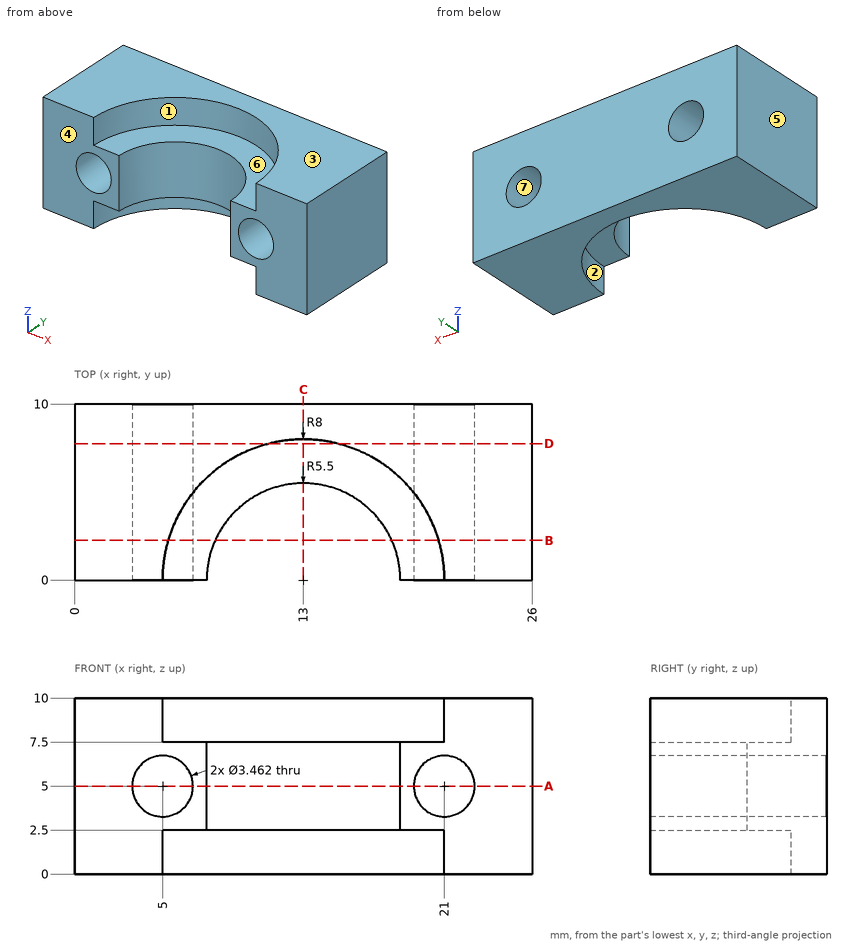
Input: dimensioned drawing with shaded views. Units: mm. Origin: part minimum x, y, z. A direction names the side the tool comes from. Give positions to 0.01 mm unless a question says otherwise; leave off trailing zeros. Write each loop counter-clockwise with the first axis right and the second up, starting at its lowest first coordinate (ties: lowest second). Pieces come first, ordered by that corner, then holes. Notation, with made-up numbers: (14, 72.25) -> (65, 72.25) arc R14 cw to (65, 93.25) -> close; hole circle Ø1 at (-3.5, -35.75). An arc over 180 degrees is marked (long way). Return JSON: item names as keys, results as strings. Group by question number.
1. Section A-A, the plane z = 5. Output: boundary loops of the cut face in (x, y).
2. Pin query (flat end, axial travel): pin 1 Ø2 at (y, z) = (8.5, 7) entering from -X; pin 2 Ø2 at (x, y) = (7.5, 1.5) entering from -Z; pin 3 Ø2 at (x, z) = (15.5, 4.5) entering from -Y. Return the tip coordinate at first contact, or that it passes through.
3. Material intervals for line 1 (Z direction, x = 21, y = 3.25); line 2 (Z direction, x = 7.75, y = 4.75); line 3 (X direction, y = 4, z = 1.25), sorted ascending. Write a range as from..to.
4. Mould query, pull axis X, two halves, no side actions, for the marked faces 4, 5, 6 and 7. Classes: +X half, -X half, draft (parallel to the pull), parting line (faces both ways), or undercut.
5. Access query for the marked faces 1, 2 and 3. Directions: +Z, -Z, +X, -X, +Y, -Y. A direction counts if a zero-diameter tool reaches every point of the face in a straight line with its end or side. Return the directions, or none.
6. Section B-B, the plane y = 2.25. Output: boundary loops of the cut face in (x, z), then the cut area to 3 significant figures.
7. Section D-D, the plane y = 7.75. Output: boundary loops of the cut face in (x, z).
8. Section C-C, the plane x = 13. Output: boundary loops of the cut face in (y, z), then the cut area to 3 significant figures.
Determined:
{
 "1": {"outline": "(0, 0) -> (3.27, 0) -> (3.27, 10) -> (0, 10) -> close; (6.73, 0) -> (7.5, 0) arc R5.5 cw to (18.5, 0) -> (19.27, 0) -> (19.27, 10) -> (6.73, 10) -> close; (22.73, 0) -> (26, 0) -> (26, 10) -> (22.73, 10) -> close"},
 "2": {"pin 1": "stops at x = 0", "pin 2": "stops at z = 2.5", "pin 3": "stops at y = 4.24"},
 "3": {"line 1": "z = 0..3.27, 6.73..10", "line 2": "z = 2.5..7.5", "line 3": "x = 0..6.07, 19.93..26"},
 "4": {"face 4": "draft", "face 5": "-X half", "face 6": "undercut", "face 7": "undercut"},
 "5": {"face 1": "+Z, -Y", "face 2": "-Z, -Y", "face 3": "+Z, +X, -X, +Y, -Y"},
 "6": {"outline": "(0, 0) -> (5.32, 0) -> (5.32, 2.5) -> (7.98, 2.5) -> (7.98, 7.5) -> (5.32, 7.5) -> (5.32, 10) -> (0, 10) -> close; (18.02, 2.5) -> (20.68, 2.5) -> (20.68, 0) -> (26, 0) -> (26, 10) -> (20.68, 10) -> (20.68, 7.5) -> (18.02, 7.5) -> close; hole circle Ø3.46 at (5, 5); hole circle Ø3.46 at (21, 5)", "area": "114 mm2"},
 "7": {"outline": "(0, 0) -> (11.02, 0) -> (11.02, 2.5) -> (14.98, 2.5) -> (14.98, 0) -> (26, 0) -> (26, 10) -> (14.98, 10) -> (14.98, 7.5) -> (11.02, 7.5) -> (11.02, 10) -> (0, 10) -> close; hole circle Ø3.46 at (5, 5); hole circle Ø3.46 at (21, 5)"},
 "8": {"outline": "(5.5, 2.5) -> (8, 2.5) -> (8, 0) -> (10, 0) -> (10, 10) -> (8, 10) -> (8, 7.5) -> (5.5, 7.5) -> close", "area": "32.5 mm2"}
}
